For this review, take the finished solid that the model builds, in its own axes (mm). Face numbers are marked on the shaded views. A direction names the side the tool comes from. Round coordinates to 2 decimals unless told otherwise and drop trailing zeros. Write each loop counter-clockwise with the first axis right and the second up, starting at its lowest first coordinate (ties: lowest second). Pieces come first, ordered by that corner, then holes. Notation, with made-up numbers: M 53.5,67 L 65.5,67 A25 cw 65.5,97 Z; hole C 29.25,-31 d1. An arc over 180 degrees is marked long. One line per question, with ' | ' between items.
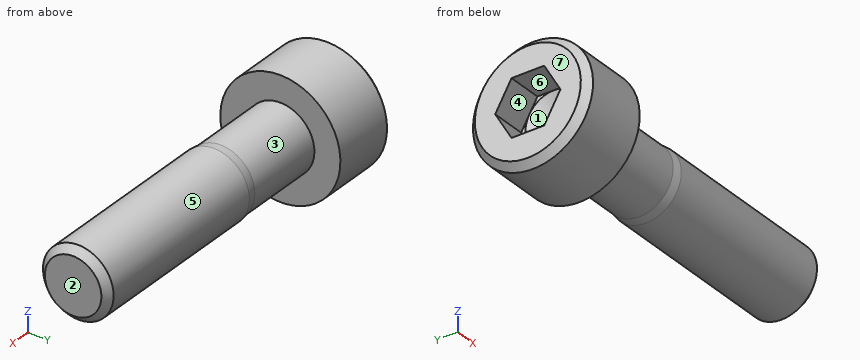
```python
from build123d import *

# Parameters (mm, degrees)
SKETCH1_W           = 5
SKETCH1_H           = 4.25
SKETCH2_R           = 2.41
BOSS_EXTRUDE1_DEPTH = 5.746788991
SKETCH3_R           = 2.41
BOSS_EXTRUDE2_DEPTH = 0.653211009
BOSS_EXTRUDE2_DRAFT = -7.844871593
SKETCH4_R           = 2.5
BOSS_EXTRUDE3_DEPTH = 13.6
CUT_EXTRUDE1_DEPTH  = 2.5
CHAMFER1_SIZE       = 0.5


with BuildPart() as part:
    # Sketch1 → Revolve1 (revolve)
    with BuildSketch(Plane(origin=(0, 0, 0), x_dir=(-1, 0, 0), z_dir=(0, 0, -1)), mode=Mode.PRIVATE) as revolve1_sk:
        with Locations((2.5, 2.125)):
            Rectangle(SKETCH1_W, SKETCH1_H)
    revolve(revolve1_sk.sketch.rotate(Axis((0, 0, 0), (-1, 0, 0)), 270), axis=Axis((0, 0, 0), (-1, 0, 0)))

    # Sketch2 → Boss-Extrude1 (add)
    with BuildSketch(Plane(origin=(0, 0, 0), x_dir=(0, 0, -1), z_dir=(1, 0, 0))):
        Circle(SKETCH2_R)
    extrude(amount=BOSS_EXTRUDE1_DEPTH)


with BuildPart() as boss_extrude2_tool:
    # Sketch3 → Boss-Extrude2 (with draft: the straight prism first)
    with BuildSketch(Plane(origin=(5.746788991, 0, 0), x_dir=(0, 0, -1), z_dir=(1, 0, 0))):
        Circle(SKETCH3_R)
    extrude(amount=BOSS_EXTRUDE2_DEPTH)
    # Boss-Extrude2: the draft: its side faces are tilted about the plane it starts from
    boss_extrude2_sides = [boss_extrude2_tool.faces().sort_by_distance(p)[0] for p in [
        (6.073394495, 0, 2.41),
    ]]
    draft(boss_extrude2_sides, Plane(origin=(5.746788991, 0, 0), x_dir=(0, 0, -1), z_dir=(1, 0, 0)), BOSS_EXTRUDE2_DRAFT)


with BuildPart() as part_1:
    add(part.part)

    # Boss-Extrude2: add boss_extrude2_tool
    add(boss_extrude2_tool.part)

    # Sketch4 → Boss-Extrude3 (add)
    with BuildSketch(Plane(origin=(6.4, 0, 0), x_dir=(0, 0, -1), z_dir=(1, 0, 0))):
        Circle(SKETCH4_R)
    extrude(amount=BOSS_EXTRUDE3_DEPTH)

    # Sketch5 → Cut-Extrude1 (cut)
    with BuildSketch(Plane.ZY.offset(5)):
        Polygon((-2, -1.154700538), (0, -2.309401077), (2, -1.154700538), (2, 1.154700538), (0, 2.309401077), (-2, 1.154700538), align=None)
    extrude(amount=-CUT_EXTRUDE1_DEPTH, mode=Mode.SUBTRACT)

    # Sketch6 → Cut-Revolve1 (revolve, cut)
    with BuildSketch(Plane.XY, mode=Mode.PRIVATE) as cut_revolve1_sk:
        Polygon((-2.5, 2), (-2.5, 0), (-1.345299462, 0), align=None)
    revolve(cut_revolve1_sk.sketch.rotate(Axis((-2.500025, 0, 0), (1, 0, 0)), 90), axis=Axis((-2.500025, 0, 0), (1, 0, 0)), mode=Mode.SUBTRACT)

    # Chamfer1
    chamfer1_edges = [part_1.edges().sort_by_distance(p)[0] for p in [
        (20, 0, 2.5),
        (-5, 0, -4.25),
    ]]
    chamfer(chamfer1_edges, length=CHAMFER1_SIZE)


solid = part_1.part
```
Item 1: To check wall thickness, follow line 1 along Y through (x, z) = (9.25, 0); line 2 along Z through (x, y) = (14.75, -1.5); line 3 along X through (y, z) = (1.25, 2.5). State the ranges of each line that lie inside material, in increasing order. Write a range as from..to.
Results:
line 1: -2.5..2.5 | line 2: -2..2 | line 3: -5..0
Item 2: Machinability: for the marked faces 5, 6 and 7, which of the approach directions +Z, -Z, +X, -X, +Y, -Y give a long, thin tool a straight path to every point of the face, cutting with its end or side? Answer none if there is none.
Results:
face 5: +X | face 6: -X | face 7: +Z, -Z, -X, +Y, -Y
Item 3: Insertion check: pin 1 Ø1.5 at (x, y) = (9.5, -1.5) entering from -Z; pin 2 Ø3 at (x, z) = (5.5, 1.5) entering from +Y; pin 3 Ø4 at (x, z) = (6, 1.5) entering from -Y. Each pin has a flat end and moves straight along its axis. Give the tip position at first contact, or say it passes through.
Results:
pin 1: z = -2.38 | pin 2: y = 2.48 | pin 3: y = -2.5
Item 4: Mouldability with a two-part tool opening along X and no side actions: class the marked faces 1, 2, 3 and 4 as +X half, -X half, draft (parallel to the pull), parting line (faces both ways), or undercut.
Results:
face 1: -X half | face 2: +X half | face 3: undercut | face 4: draft
Item 5: Take a section at B-B (x = 1.75). Write out the cut boundary in (y, z).
Results:
outline: C 0,0 d4.82
Item 6: Take a section at A-A (x = 10.75). Write out the cut boundary in (y, z).
Results:
outline: C 0,0 d5
